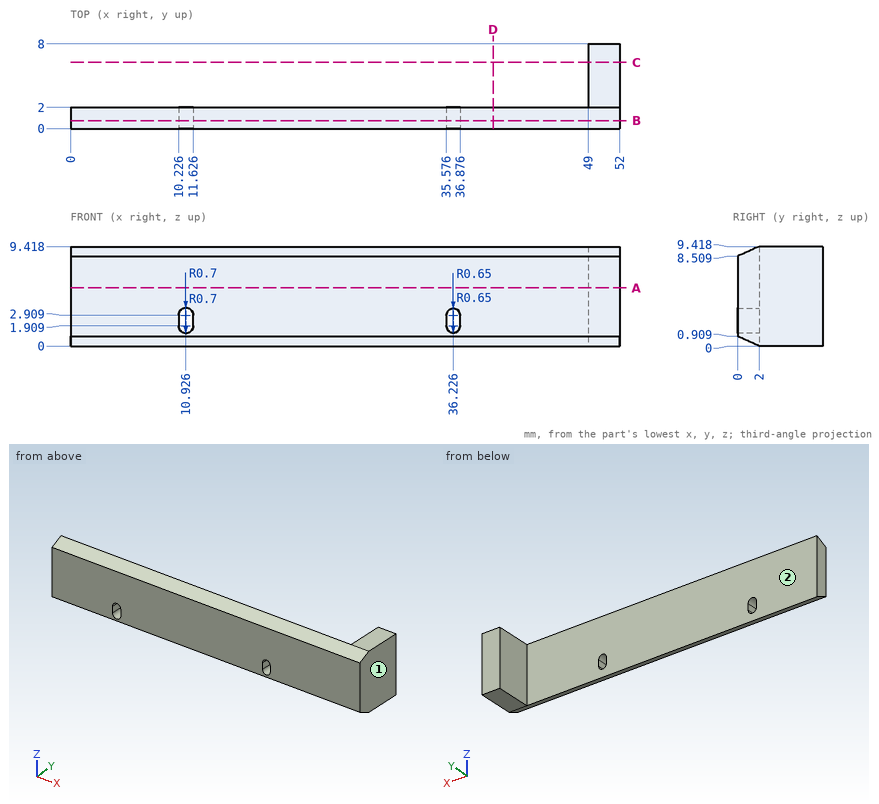
Input: dimensioned drawing with shaded views. Units: mm. Origin: part minimum x, y, z. A direction names the side the tool comes from. Round coordinates to 2 decimals unless told otherwise and drop trailing zeros. Loops run counter-clockwise (first coordinate to the right, second up) from the corner with the lowest first, then second, coordinate; pieces in that order, holes last. Notation, with made-up numbers: (39.5, 47.5) -> (93.5, 47.5) arc R28 ccw to (93.5, 77.5) -> close; hole circle Ø8 at (40.25, 73). An arc over 180 degrees is marked (long way). Answer as a JSON object with one key per item and string values. Group by question number.
Q1. Section query B-B (y = 0.75). Output: boundary loops of the cut face in (x, z), plus the area to 3 significant figures.
Q2. Access query for the marked faces 1 and 2. Directions: +Z, -Z, +X, -X, +Y, -Y. A direction counts if a zero-diameter tool reaches every point of the face in a straight line with its end or side. Return the directions, or none.
Q3. Ray query, line 1 (X direction, y = 4, z = 4.5); line 2 (X direction, y = 0.5, z = 3.25) (1 decimal); line 3 (Y direction, x = 29, z = 6.5). Return the intervals inside material, ascending. Write a range as from..to.
Q4. Section query D-D (x = 40). Output: boundary loops of the cut face in (y, z).
Q5. Section query A-A (z = 5.5). Output: boundary loops of the cut face in (x, y).
Q6. Contact query for flat-ended pins moving along their axis: P1, Ø2, axis at x = 16, z = 2.5, coming from the +Y side; P2, Ø1.8, axis at y = 5, z = 3.5, coming from the -X side. Output: stop coordinate, or through.
Q7. Section query C-C (y = 6.25). Output: boundary loops of the cut face in (x, z).
Completed:
{
 "1": {"outline": "(0, 0.57) -> (52, 0.57) -> (52, 8.85) -> (0, 8.85) -> close; hole (10.23, 1.91) arc R0.7 ccw to (11.63, 1.91) -> (11.63, 2.91) arc R0.7 ccw to (10.23, 2.91) -> close; hole (35.58, 1.91) arc R0.65 ccw to (36.88, 1.91) -> (36.88, 2.91) arc R0.65 ccw to (35.58, 2.91) -> close", "area": "425 mm²"},
 "2": {"face 1": "+Z, -Z, +X, +Y, -Y", "face 2": "+Z, -Z, -X, +Y"},
 "3": {"line 1": "49..52", "line 2": "0..10.3, 11.5..35.7, 36.8..52", "line 3": "0..2"},
 "4": {"outline": "(0, 0.91) -> (2, 0) -> (2, 9.42) -> (0, 8.51) -> close"},
 "5": {"outline": "(0, 0) -> (52, 0) -> (52, 8) -> (49, 8) -> (49, 2) -> (0, 2) -> close"},
 "6": {"P1": "y = 2", "P2": "x = 49"},
 "7": {"outline": "(49, 0) -> (52, 0) -> (52, 9.42) -> (49, 9.42) -> close"}
}
